from build123d import *

# Parameters (mm, degrees)
PAD_DEPTH            = 42.5
SKETCH001_W          = 11
SKETCH001_H          = 12
POCKET_DEPTH         = 19.001
POCKET001_DEPTH      = 229.0486136499
SKETCH003_W          = 21
SKETCH003_H          = 24
POCKET002_DEPTH      = 19.001
POCKET002_DEPTH_BACK = 2.001
POCKET003_DEPTH      = 26.5
SKETCH006_R          = 2.45
PAD001_DEPTH         = 3.5
SKETCH007_R          = 1.5
PAD002_DEPTH         = 3.5
SKETCH008_R          = 4.25
PAD003_DEPTH         = 7
SKETCH009_W          = 24
SKETCH009_H          = 5.7855610815
POCKET004_DEPTH      = 38.3792032733
SKETCH010_W          = 24
SKETCH010_H          = 3.7173874083
POCKET005_DEPTH      = 23.1222095644
SKETCH011_W          = 2
SKETCH011_H          = 4
POCKET006_DEPTH      = 2
CHAMFER_SIZE         = 0.5
FILLET_R             = 8


with BuildPart() as part:
    # Sketch → Pad (new body, symmetric)
    with BuildSketch(Plane.YZ):
        with BuildLine():
            Line((23.6132486541, 0), (36.6132486541, 0))
            Line((36.6132486541, 0), (39.5, 5))
            Line((39.5, 5), (39.5, 14.5))
            ThreePointArc((39.5, 14.5), (35, 19), (30.5, 14.5))
            Line((30.5, 14.5), (30.5, 8.5))
            ThreePointArc((27.5, 5.5), (29.6213203436, 6.3786796564), (30.5, 8.5))
            Line((27.5, 5.5), (23.5, 5.5))
            Line((23.5, 5.5), (16.5717967697, 9.5))
            ThreePointArc((16.5717967697, 9.5), (0.731487802, 9.2160988481), (-14.1535861905, 3.7911048117))
            Line((-18.5, 4.5574948357), (-14.1535861905, 3.7911048117))
            Line((-16.6188892117, -0.6108145787), (-18.5, 4.5574948357))
            Line((-8.7404271876, -2), (-16.6188892117, -0.6108145787))
            ThreePointArc((23.6132486541, 0), (7.1909178254, 2.97129898), (-8.7404271876, -2))
        make_face()
    extrude(amount=PAD_DEPTH, both=True)

    # Sketch001 (on Face1 of Pad) → Pocket (cut, through all)
    with BuildSketch(Plane.YX):
        with Locations((34, -1.5)):
            Rectangle(SKETCH001_W, SKETCH001_H)
    extrude(amount=-POCKET_DEPTH, mode=Mode.SUBTRACT)

    # Sketch002 (on Face1 of Pocket) → Pocket001 (cut, through all)
    with BuildSketch(Plane.YX):
        Polygon((0, 42.5), (39.5, 42.5), (39.5, 14), (27.5, 14), (25, 16), (0, 16), align=None)
    pocket001 = extrude(amount=-POCKET001_DEPTH, mode=Mode.SUBTRACT)

    # Mirrored: Pocket001 across YZ
    add(pocket001.mirror(Plane.YZ), mode=Mode.SUBTRACT)

    # Sketch003 (on Face1 of Mirrored) → Pocket002 (cut, two sides)
    with BuildSketch(Plane.YX) as pocket002_sk:
        with Locations((5, 0)):
            Rectangle(SKETCH003_W, SKETCH003_H)
    extrude(amount=-POCKET002_DEPTH, mode=Mode.SUBTRACT)
    extrude(pocket002_sk.sketch, amount=POCKET002_DEPTH_BACK, mode=Mode.SUBTRACT)

    # Sketch004 (on Face28 of Pocket002) → Pocket003 (cut)
    with BuildSketch(Plane.YZ.offset(42.5)):
        Polygon((0, 9.0743034734), (0, -11.3506822755), (-19.0919866044, 9.0743034734), align=None)
    pocket003 = extrude(amount=-POCKET003_DEPTH, mode=Mode.SUBTRACT)

    # Mirrored001: Pocket003 across YZ
    add(pocket003.mirror(Plane.YZ), mode=Mode.SUBTRACT)

    # Sketch006 (on Face9 of Mirrored001) → Pad001 (join)
    with BuildSketch(Plane.YZ.offset(14)):
        with Locations((35, 14.5)):
            Circle(SKETCH006_R)
    extrude(amount=PAD001_DEPTH)

    # Sketch007 (on Face4 of Pad001) → Pad002 (join)
    with BuildSketch(Plane(origin=(-14, 0, 0), x_dir=(0, 1, 0), z_dir=(-1, 0, 0))):
        with Locations((35, -14.5)):
            Circle(SKETCH007_R)
    extrude(amount=PAD002_DEPTH)

    # Sketch008 (on Face6 of Pad002) → Pad003 (join)
    with BuildSketch(Plane.YZ.offset(-7.5)):
        with Locations((35, 14.5)):
            Circle(SKETCH008_R)
    extrude(amount=PAD003_DEPTH)

    # Sketch009 (on DatumPlane) → Pocket004 (cut, through all)
    with BuildSketch(Plane(origin=(4.6666666667, 24.8333333333, 3.6666666667), x_dir=(-1, 0, 0), z_dir=(0, 0.8087360843, 0.5881716977))):
        with Locations((4.6666666667, 7.4335939838)):
            Rectangle(SKETCH009_W, SKETCH009_H)
    extrude(amount=-POCKET004_DEPTH, mode=Mode.SUBTRACT)

    # Sketch010 (on DatumPlane) → Pocket005 (cut, through all)
    with BuildSketch(Plane(origin=(-5.3333333333, -6.5801423959, -0.8458036702), x_dir=(1, 0, 0), z_dir=(0, -0.4712379677, 0.8820061099))):
        with Locations((5.3333333333, 3.0833364632)):
            Rectangle(SKETCH010_W, SKETCH010_H)
    extrude(amount=POCKET005_DEPTH, mode=Mode.SUBTRACT)

    # Sphere → Sphere (revolve, cut)
    with BuildSketch(Plane(origin=(0, -12, 27), x_dir=(0, 0, 1), z_dir=(-1, 0, 0))):
        with BuildLine():
            ThreePointArc((0, -25), (25, 0), (0, 25))
            Line((0, 25), (0, -25))
        make_face()
    revolve(axis=Axis((0, -12, 27), (0, 1, 0)), mode=Mode.SUBTRACT)

    # Sketch011 (on Face1 of Sphere) → Pocket006 (cut)
    with BuildSketch(Plane(origin=(0, -12, 0), x_dir=(-1, 0, 0), z_dir=(0, 0, -1))):
        with Locations((5.5, 38.5)):
            Rectangle(SKETCH011_W, SKETCH011_H)
    extrude(amount=-POCKET006_DEPTH, mode=Mode.SUBTRACT)

    # Chamfer
    chamfer_edges = [part.edges().sort_by_distance(p)[0] for p in [
        (17.5, 32.55, 14.5),
        (-0.5, 30.75, 14.5),
        (-17.5, 33.5, 14.5),
    ]]
    chamfer(chamfer_edges, length=CHAMFER_SIZE)

    # Fillet
    fillet_edges = [part.edges().sort_by_distance(p)[0] for p in [
        (16, -11.447007, 0.895552),
        (-16, -11.447007, 0.895552),
    ]]
    fillet(fillet_edges, radius=FILLET_R)


solid = part.part
Part model, mm, in its own coordinate system. A direction names the side the tool comes from. Coordinates: 2 decimals unless noted, no trailing zeros. Write each loop counter-clockwise with the first axis right and the second up, starting at its lowest first coordinate (ties: lowest second). Pieces come first, ordered by that corner, then holes. Notation, with made-up numbers: M -15,-23 L -10,-23 A20 cw -10,10 Z; hole C 36,0.25 d7. An arc over 180 degrees is marked long. Return JSON: item names as keys, results as strings.
1. Probe L1, parallel to X at y = 32, z = 6.25; L2, parallel to X at y = 8.5, z = 9.5; L3, parallel to Y at x = -27.5, z = 3. List the from-to ranges inside material, lowest first.
Determined:
{"L1": "-14 to -7.5, 4.5 to 14", "L2": "-16 to -12, 12 to 16", "L3": "-17.93 to -13.41"}
2. Flat gauge pins, fed straight in: pin 1 Ø5 at (y, z) = (16.5, 6) entering from -X; pin 2 Ø1.5 at (y, z) = (28, 8) entering from +X; pin 3 Ø4.5 at (y, z) = (35.5, 14) entering from +X; pin 4 Ø2 at (x, y) = (4, 25) entering from +Z. Where does each tip first touch, or does it go through?
Determined:
{"pin 1": "x = -16", "pin 2": "through", "pin 3": "x = 17.5", "pin 4": "z = 5.5"}
3. Saw through at D-D, the plane x = -19. Write the cut outline in (y, z), then the cut area to 3 significant figures.
Determined:
{"outline": "M -18.5,4.56 L -16.62,-0.61 L -8.74,-2 A35 cw -7.17,-1.11 L -12.56,4.65 A48 ccw -14.15,3.79 Z", "area": "43.4 mm²"}
4. Saw through at B-B, the plane x = -2.5. Write the cut outline in (y, z), then the cut area to 3 significant figures.
Determined:
{"outline": "M -17.87,2.83 L -16.62,-0.61 L -8.74,-2 A35 cw -5.5,-0.27 L -7.05,2.62 A24.87 cw Z; M 15.5,2.49 A35 cw 23.61,0 L 28.5,0 L 28.5,5.67 A3 cw 27.5,5.5 L 23.5,5.5 L 21.34,6.74 Z; C 35,14.5 d8.5", "area": "152 mm²"}
5. Saw through at A-A, the plane y = 35. Write the cut outline in (x, z), then the cut area to 3 significant figures.
Determined:
{"outline": "M -17.5,13.5 L -17,13 L -14,13 L -14,0 L -7.5,0 L -7.5,10.25 L -1,10.25 L -0.5,10.75 L -0.5,18.25 L -1,18.75 L -7.5,18.75 L -7.5,19 L -14,19 L -14,16 L -17,16 L -17.5,15.5 Z; M 4.5,0 L 14,0 L 14,12.05 L 17,12.05 L 17.5,12.55 L 17.5,16.45 L 17,16.95 L 14,16.95 L 14,19 L 4.5,19 Z", "area": "390 mm²"}
6. Pull direction X, two halves, no side cores. Call faces 4 (the face through (9, 30.5, 12)), 5 (the face through (42.5, -15, 1)), 6 (the face through (4.5, 34, 9)): pulls with the +X half, pulls with the -X half, needs draft (parallel to the pull), parting line crosses it, or undercut.
Determined:
{"face 4": "needs draft", "face 5": "pulls with the +X half", "face 6": "undercut"}
7. Saw through at C-C, the plane y = 8.5. Write the cut outline in (x, z), then the cut area to 3 significant figures.
Determined:
{"outline": "M -16,3.03 L -12,3.03 L -12,10.01 L -16,10.01 Z; M 12,3.03 L 16,3.03 L 16,10.01 L 12,10.01 Z", "area": "55.9 mm²"}
8. 3-axis set-ups, long thin cutter, end or side, ignore diameter. For faces 1 (the face through (-4.5, 26, 1)), 2 (the face through (-0.5, 35, 15)), 3 (the face through (12, 6, 6)): which of +Z, -Z, +X, -X, +Y, -Y reach the whole face in a straight line?
Determined:
{"face 1": "-Z, +Y", "face 2": "+Z, -Z, +Y, -Y", "face 3": "+Z"}
